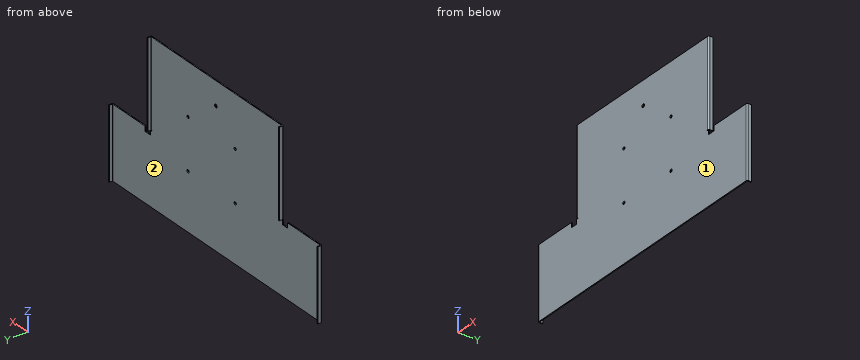
```python
from build123d import *

# Parameters (mm, degrees)
SM_BASE_FLANGE_1_DEPTH   = 3
SM_START                 = 216.5
SM_EDGE_FLANGE_1_DEPTH   = 266.233197448
SM_EDGE_FLANGE_1_2_DEPTH = 216.5
SM_START_2               = 218
SM_EDGE_FLANGE_1_3_DEPTH = 264.733197448
SM_EDGE_FLANGE_1_4_DEPTH = 218
SM_START_3               = -1
SM_EDGE_FLANGE_1_5_DEPTH = 4.74
SKETCH_14_R              = 5
SKETCH_14_R_2            = 4.25
CUT_EXTRUDE_1_DEPTH      = 10


with BuildPart() as part:
    # Базовая кромка1: sheet metal written as solids
    # Sketch 1 → Базовая кромка1 (new body)
    with BuildSketch(Plane(origin=(0, 0, 0), x_dir=(1, 0, 0), z_dir=(0, 1, 0))):
        Polygon((-410, 0), (0, 0), (0, -482.733197448), (-259.163690552, -482.733197448), (-259.163690552, -203), (-279.163690552, -203), (-279.163690552, -218), (-410, -218), align=None)
    extrude(amount=SM_BASE_FLANGE_1_DEPTH)

    # Ребро-кромка1: read off the stored shape, not the designer's step
    # Ребро-кромка1 outline → Ребро-кромка1 (cut)
    with BuildSketch(Plane.XY.offset(SM_START)):
        with BuildLine():
            ThreePointArc((-255.423690552, 0), (-257.792234409, 0.845591597), (-259.089751108, 3))
            Line((-259.089751108, 3), (-259.163690552, 3))
            Line((-259.163690552, 3), (-259.163690552, 0))
            Line((-259.163690552, 0), (-255.423690552, 0))
        make_face()
        with BuildLine():
            Line((-410, 0), (-406.26, 0))
            ThreePointArc((-406.26, 0), (-408.628543857, 0.845591597), (-409.926060556, 3))
            Line((-409.926060556, 3), (-410, 3))
            Line((-410, 3), (-410, 0))
        make_face()
    extrude(amount=SM_EDGE_FLANGE_1_DEPTH, mode=Mode.SUBTRACT)

    # Sm Edge Flange 1 2 outline → Sm Edge Flange 1 2 (cut)
    with BuildSketch(Plane.XY):
        with BuildLine():
            Line((-410, 0), (-406.26, 0))
            ThreePointArc((-406.26, 0), (-408.628543857, 0.845591597), (-409.926060556, 3))
            Line((-409.926060556, 3), (-410, 3))
            Line((-410, 3), (-410, 0))
        make_face()
    extrude(amount=SM_EDGE_FLANGE_1_2_DEPTH, mode=Mode.SUBTRACT)

    # Sm Edge Flange 1 3 outline → Sm Edge Flange 1 3 (add)
    with BuildSketch(Plane.XY.offset(SM_START_2)):
        with BuildLine():
            Line((-259.163690552, 13), (-259.163690552, 3.74))
            ThreePointArc((-259.163690552, 3.74), (-259.145159783, 3.368157614), (-259.089751108, 3))
            Line((-259.089751108, 3), (-255.423690552, 3))
            ThreePointArc((-255.423690552, 3), (-255.94694957, 3.216740982), (-256.163690552, 3.74))
            Line((-256.163690552, 3.74), (-256.163690552, 13))
            Line((-256.163690552, 13), (-259.163690552, 13))
        make_face()
    extrude(amount=SM_EDGE_FLANGE_1_3_DEPTH)

    # Sm Edge Flange 1 4 outline → Sm Edge Flange 1 4 (add)
    with BuildSketch(Plane.XY):
        with BuildLine():
            Line((-409.926060556, 3), (-406.26, 3))
            ThreePointArc((-406.26, 3), (-406.783259018, 3.216740982), (-407, 3.74))
            Line((-407, 3.74), (-407, 13))
            Line((-407, 13), (-410, 13))
            Line((-410, 13), (-410, 3.74))
            ThreePointArc((-410, 3.74), (-409.981469231, 3.368157614), (-409.926060556, 3))
        make_face()
    extrude(amount=SM_EDGE_FLANGE_1_4_DEPTH)

    # Sm Edge Flange 1 5 outline → Sm Edge Flange 1 5 (cut)
    with BuildSketch(Plane(origin=(0, 0, 0), x_dir=(1, 0, 0), z_dir=(0, 1, 0)).offset(SM_START_3)):
        with BuildLine():
            Line((-260, -218), (-253.923690552, -218))
            ThreePointArc((-253.923690552, -218), (-253.173690552, -217.25), (-253.923690552, -216.5))
            Line((-253.923690552, -216.5), (-260, -216.5))
            Line((-260, -216.5), (-260, -218))
        make_face()
    extrude(amount=SM_EDGE_FLANGE_1_5_DEPTH, mode=Mode.SUBTRACT)

    # Зеркальное отражение1: part across plane


with BuildPart() as part_1:
    add(part.part)
    add(part.part.mirror(Plane(origin=(0, 3, 0), x_dir=(0, 0, 1), z_dir=(-1, 0, 0))))

    # Эскиз14 → Вырез-Вытянуть1 (cut)
    with BuildSketch(Plane(origin=(0, 3, 0), x_dir=(1, 0, 0), z_dir=(0, 1, 0))):
        with Locations(Location((2.5, -410.733197448, 0), (0, 0, 270))):
            Circle(SKETCH_14_R)
        with Locations(Location((111.6195, -172.648893261, 0), (0, 0, 270))):
            Circle(SKETCH_14_R_2)
        with Locations(Location((111.6195, -326.461239213, 0), (0, 0, 270))):
            Circle(SKETCH_14_R_2)
        with Locations(Location((-73.3805, -326.461239213, 0), (0, 0, 270))):
            Circle(SKETCH_14_R_2)
        with Locations(Location((-73.3805, -172.648893261, 0), (0, 0, 270))):
            Circle(SKETCH_14_R_2)
    extrude(amount=-CUT_EXTRUDE_1_DEPTH, mode=Mode.SUBTRACT)


solid = part_1.part
```
Source: CAD feature listing. Evaluate the final solid. Frame: model axes, mm. Face numbers are marked on the shaded views. Round coordinates to 2 decimals unless told otherwise and drop trailing zeros. Order: outer loops, then holes, each group sorted by start corner. A loop starts at its lowest first (then second) coordinate and runs counter-clockwise, first axis right, second up. Notation, with made-up numbers: (12, 6) -> (20, 6) arc R20 cw to (20, 28) -> close; hole circle Ø3 at (-9.5, 15). An arc over 180 degrees is marked (long way). One line per item, written item: value. Start each with the question number.
Q1. Draft query along X for the marked faces 1 and 2. Return one class per face: pulls with the +X half, pulls with the -X half, needs draft (parallel to the pull), parting line crosses it, or undercut.
Q2. Section query B-B (z = 78). Return the cut outline in (x, y).
Q3. Section query C-C (x = 84). Return the cut outline in (y, z).
Q4. Material intervals for probe 1 along X at (y, z) = (5.5, 181); probe 2 along X at (y, z) = (11.5, 457); probe 3 along Y at (x, z) = (205.5, 265.5), sorted ascending.
Q5. Section query D-D (z = 284). Return the cut outline in (x, y).
Q6. Section query A-A (y = 11). Return the cut outline in (x, z).
Q7. Pin query (flat end, axial travel): pin 1 (0.9 mm diameter, centred on y = 2, z = 209.5, fed in from -X); pin 2 (13.5 mm diameter, centred on x = 111.62, z = 326.46, fed in from +Y); pin 3 (7.5 mm diameter, centred on y = 6.5, z = 302, fed in from -X). Return the tip coordinate at first contact, or that it passes through.
Findings below:
1. face 1: needs draft
1. face 2: undercut
2. outline: (-410, 3.74) arc R3.74 ccw to (-406.26, 0) -> (406.26, 0) arc R3.74 ccw to (410, 3.74) -> (410, 13) -> (407, 13) -> (407, 3.74) arc R0.74 cw to (406.26, 3) -> (-406.26, 3) arc R0.74 cw to (-407, 3.74) -> (-407, 13) -> (-410, 13) -> close
3. outline: (0, 0) -> (3, 0) -> (3, 482.73) -> (0, 482.73) -> close
4. probe 1: -410 to -407, 407 to 410
4. probe 2: -259.16 to -256.16, 256.16 to 259.16
4. probe 3: 0 to 3
5. outline: (-259.16, 3.74) arc R3.74 ccw to (-255.42, 0) -> (255.42, 0) arc R3.74 ccw to (259.16, 3.74) -> (259.16, 13) -> (256.16, 13) -> (256.16, 3.74) arc R0.74 cw to (255.42, 3) -> (-255.42, 3) arc R0.74 cw to (-256.16, 3.74) -> (-256.16, 13) -> (-259.16, 13) -> close
6. outline: (-410, 0) -> (-407, 0) -> (-407, 218) -> (-410, 218) -> close; (-259.16, 218) -> (-256.16, 218) -> (-256.16, 482.73) -> (-259.16, 482.73) -> close; (256.16, 218) -> (259.16, 218) -> (259.16, 482.73) -> (256.16, 482.73) -> close; (407, 0) -> (410, 0) -> (410, 218) -> (407, 218) -> close
7. pin 1: x = -409.77
7. pin 2: y = 3
7. pin 3: x = -259.16
